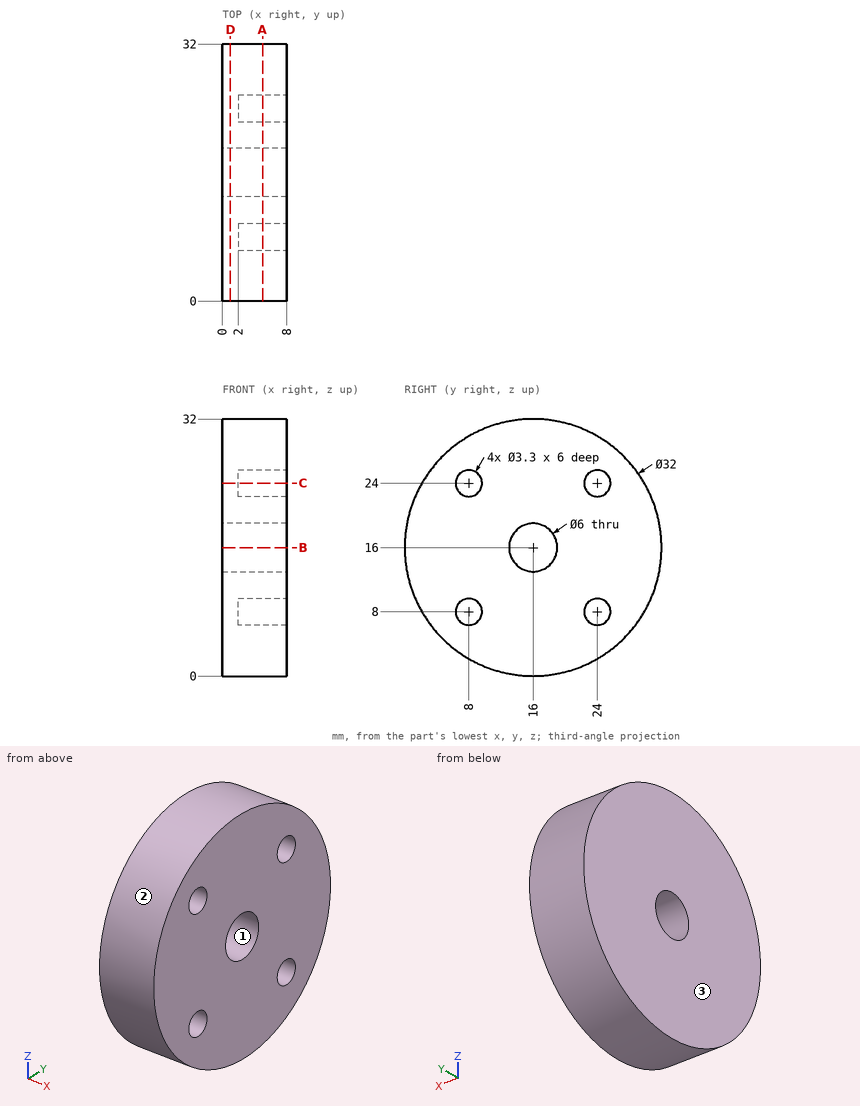
Part print with two shaded views. Sizes in mm from the minimum x, y, z corner. Give positions to 0.01 mm unless a question says otherwise; leave off trailing zeros. Write each loop counter-clockwise with the first axis right and the second up, starting at its lowest first coordinate (ties: lowest second). Pieces come first, ordered by that corner, then holes.
1) Two-plate mould, pull along Y, no slides. Class the marked faces 1, 2 and 3: released by +Y, released by -Y, zero draft, split by the parting line, or undercut.
Resolved:
face 1: undercut
face 2: split by the parting line
face 3: zero draft
2) Cut at B-B on z = 16. Write the cut outline in (x, y), then the cut area to 3 significant figures.
Resolved:
outline: (0, 0) - (8, 0) - (8, 13) - (0, 13) - close; (0, 19) - (8, 19) - (8, 32) - (0, 32) - close
area: 208 mm2
3) Probe L1, parallel to Y at x = 5.55, z = 8; L2, parallel to Z at x = 5.25, y = 25.5; L3, parallel to Z at x = 5.75, y = 7. List the from-to ranges inside material, lowest first.
Resolved:
L1: y = 2.14 to 6.35, 9.65 to 22.35, 25.65 to 29.86
L2: z = 3.13 to 7.31, 8.69 to 23.31, 24.69 to 28.87
L3: z = 2.77 to 6.69, 9.31 to 22.69, 25.31 to 29.23
4) Pin check, flat tips, straight feed: pin 1 (1.5 mm diameter, centred on y = 17.5, z = 16, fed in from +X); pin 2 (2.5 mm diameter, centred on y = 8.5, z = 24, fed in from +X); pin 3 (1.5 mm diameter, centred on x = 3.5, y = 27, fed in from -Z); pin 4 (1 mm diameter, centred on x = 1.5, z = 24.5, fed in from +Y). Stop position of each tip, or through.
Resolved:
pin 1: passes through
pin 2: stops at x = 8
pin 3: stops at z = 3.71
pin 4: stops at y = 29.86
5) Cut at A-A on x = 5. Write the cut outline in (y, z), then the cut area to 3 significant figures.
Resolved:
outline: circle Ø32 at (16, 16); hole circle Ø3.3 at (8, 8); hole circle Ø3.3 at (8, 24); hole circle Ø6 at (16, 16); hole circle Ø3.3 at (24, 8); hole circle Ø3.3 at (24, 24)
area: 742 mm2
6) Cut at D-D on x = 1. Write the cut outline in (y, z), then the cut area to 3 significant figures.
Resolved:
outline: circle Ø32 at (16, 16); hole circle Ø6 at (16, 16)
area: 776 mm2
7) Cut at C-C on z = 24. Write the cut outline in (x, y), then the cut area to 3 significant figures.
Resolved:
outline: (0, 2.14) - (8, 2.14) - (8, 6.35) - (2, 6.35) - (2, 9.65) - (8, 9.65) - (8, 22.35) - (2, 22.35) - (2, 25.65) - (8, 25.65) - (8, 29.86) - (0, 29.86) - close
area: 182 mm2
